Source: CAD feature listing. Evaluate the final solid. Frame: model axes, mm. A direction names the side the tool comes from. Coordinates: 2 decimals unless noted, no trailing zeros. One line per question, with ' | ' between items. Start each with the question number.
(1) Line query: line 1 along X through (y, z) = (-9.5, -20); line 2 along Y through (x, z) = (0, 23.55). Output: solid intervals per line, ascending.
(2) Section A-A (z = 4). Count the separate pieces of the cut face and the enclosed holes in it, then the cut area to 3 significant figures.
(3) Draft query along X for faces 1 (the cylindrical face through (-20.864, 16.323, 16.204)), 2 (the flat face through (-17, 11, -25)). Return one class per face: +X half, -X half, draft (parallel to the pull), parting line (faces both ways), or undercut.
(4) Contact query for a flat-ended pin moving along its axis: P1, Ø10, axis at x = -5.5, z = 13.5, coming from the +Y side. Output: stop coordinate, or through.
(5) Access query for faces 3 (the flat face through (-17, 25, 11)), 4 (the cylindrical face through (16.323, -20.895, 16.204)). Directions: +Z, -Z, +X, -X, +Y, -Y. A direction counts if a zero-diameter tool reaches every point of the face in a straight line with its end or side. Return the directions, or none.
from build123d import *

# Parameters (mm, degrees)
F0_W      = 50
F0_H      = 50
F1_DEPTH  = 25
F2_R      = 20
F3_DEPTH  = 50.001
F4_R      = 20
F5_DEPTH  = 50.001
F6_R      = 20
F7_DEPTH  = 50.001
F8_R      = 23
F9_DEPTH  = 23
F10_R     = 23
F11_DEPTH = 23
F12_R     = 23
F13_DEPTH = 23


with BuildPart() as f1:
    # F0 (on Top) → F1 (new body, symmetric)
    with BuildSketch(Plane.XY):
        Rectangle(F0_W, F0_H)
    extrude(amount=F1_DEPTH, both=True)

    # F2 (on face) → F3 (cut, through all)
    with BuildSketch(Plane(origin=(0, 25, 0), x_dir=(-1, 0, 0), z_dir=(0, 1, 0))):
        Circle(F2_R)
    extrude(amount=-F3_DEPTH, mode=Mode.SUBTRACT)

    # F4 (on face) → F5 (cut, through all)
    with BuildSketch(Plane(origin=(-25, 0, 0), x_dir=(0, -1, 0), z_dir=(-1, 0, 0))):
        Circle(F4_R)
    extrude(amount=-F5_DEPTH, mode=Mode.SUBTRACT)

    # F6 (on face) → F7 (cut, through all)
    with BuildSketch(Plane.XY.offset(25)):
        Circle(F6_R)
    extrude(amount=-F7_DEPTH, mode=Mode.SUBTRACT)

    # F8 (on Top) → F9 (cut, symmetric)
    with BuildSketch(Plane.XY):
        Circle(F8_R)
    extrude(amount=F9_DEPTH, both=True, mode=Mode.SUBTRACT)

    # F10 (on Right) → F11 (cut, symmetric)
    with BuildSketch(Plane.YZ):
        Circle(F10_R)
    extrude(amount=F11_DEPTH, both=True, mode=Mode.SUBTRACT)

    # F12 (on Front) → F13 (cut, symmetric)
    with BuildSketch(Plane.XZ):
        Circle(F12_R)
    extrude(amount=F13_DEPTH, both=True, mode=Mode.SUBTRACT)


solid = f1.part
Response values:
1) line 1: x = -25 to -23, 23 to 25 | line 2: y = -25 to -20, 20 to 25
2) separate pieces: 4 | enclosed holes: 0 | area: 71.0 mm²
3) face 1: undercut | face 2: draft
4) P1: passes through
5) face 3: +Z, -Z, +X, -X, +Y | face 4: none
